Autodesk Inventor part; units mm, degrees
ref_plane "Work Plane1" through (-3.0381, -3.0381, 30.2492) normal (0, 0, -1) x (0, 1, 0)
ref_plane "Work Plane2" through (-3.0898, -3.0898, 32.8492) normal (0, 0, -1) x (0.0301, 0.9995, 0)
ref_plane "YZ Plane" through (0, 0, 0) normal (1, 0, 0) x (0, 1, 0)
sketch "Sketch2" plane through (0, 0, 0) normal (0, 0, 1) x (1, 0, 0)
  circle A0 centre (0, 0) radius 3
  dimension "d0" = 6
ref_plane "Work Plane1" through (-3.0381, -3.0381, 30.2492) normal (0, 0, -1) x (0, 1, 0)
ref_plane "Work Plane2" through (-3.0898, -3.0898, 32.8492) normal (0, 0, -1) x (0.0301, 0.9995, 0)
extrude "Extrusion1" add sketch "Sketch2" along normal up to surface (32.8492 mm away)
sketch "Sketch3" plane through (0, 0, 32.8492) normal (0, 0, 1) x (1, 0, 0)
  point P0 (0, 0)
  point P1 (0, 0)
hole "Hole1" at (0, 0, 32.8492) direction (0, 0, -1) diameter 3.242 depth 10
sketch "Sketch4" plane through (0, 0, 0) normal (0, 0, -1) x (-1, 0, 0)
  circle A0 centre (0, 0) radius 1.621
  point P0 (0, 0)
hole "Hole2" at (0, 0, 0) direction (0, 0, 1) diameter 3.242 depth 10
properties part number "GEARBOX STANDOFFS"
For this review, take the finished solid that the model builds, in its own axes (mm). A direction names the side the tool comes from. Coordinates: 2 decimals unless noted, no trailing zeros. Order: outer loops, then holes, each group sorted by start corner. A loop starts at its lowest first (then second) coordinate and runs counter-clockwise, first axis right, second up. Notation, with made-up numbers: (-25, 77) -> (17, 77) arc R9 ccw to (17, 89) -> close; hole circle Ø5 at (81, -21.5). An arc over 180 degrees is marked (long way). Use CSV: the item, a comma, the result in double quotes. Start each with the question number.
Item 1: Draft analysis for pull direction Y (two halves, no side actions). For faces 1 (the face through (-3, 0, 16)), 2 (the face through (1.3, -1.3, 32.849)), 3 (the face through (1.438, 0.748, 5.07)), state which applies: pulls with the +Y half, pulls with the -Y half, needs draft (parallel to the pull), parting line crosses it, or undercut.
Item 2: Insertion check: pin 1 (1 mm diameter, centred on x = 0.5, y = 0, fed in from -Z); pin 2 (1.5 mm diameter, centred on x = 0.5, y = -0.5, fed in from +Z); pin 3 (1 mm diameter, centred on y = -1.5, z = 12.5, fed in from -X). Each pin has a flat end and moves straight along its axis. Give the tip position at first contact, or say it passes through.
Item 3: We need section C-C, the plane z = 8. Give the boundary of the cut face in (x, y).
Item 4: We need section A-A, the plane y = 0. Give the boundary of the cut face in (x, z), then the cut area to 3 significant figures.
Item 5: For faces 4 (the face through (1.3, -1.3, 0)), 5 (the face through (1.438, -0.748, 27.779)), 6 (the face through (0, 0, 10)), list the 3-axis set-ups (+Z, -Z, +X, -X, +Y, -Y) from which the entire face can be reached by the end or side of a thin tool; tool diameter is ignored.
Item 6: Wall thickness on probe 1 along X at (y, z) = (-0.05, 28.5); probe 2 along Z at (x, y) = (1, 0.75): over which ranges is each line inside the solid? List them lowest first.
Item 7: We need section D-D, the plane x = -2.1. Give the boundary of the cut face in (y, z), then the cut area to 3 significant figures.
Derived:
1,face 1,"parting line crosses it"
1,face 2,"needs draft"
1,face 3,"undercut"
2,pin 1,"stops at z = 10"
2,pin 2,"stops at z = 22.85"
2,pin 3,"stops at x = -2.83"
3,outline,"circle Ø6 at (0, 0); hole circle Ø3.24 at (0, 0)"
4,outline,"(-3, 0) -> (-1.62, 0) -> (-1.62, 10) -> (1.62, 10) -> (1.62, 0) -> (3, 0) -> (3, 32.85) -> (1.62, 32.85) -> (1.62, 22.85) -> (-1.62, 22.85) -> (-1.62, 32.85) -> (-3, 32.85) -> close"
4,area,"132 mm^2"
5,face 4,"-Z, +X, -X, +Y, -Y"
5,face 5,"+Z"
5,face 6,"-Z"
6,probe 1,"x = -3 to -1.62, 1.62 to 3"
6,probe 2,"z = 10 to 22.85"
7,outline,"(-2.14, 0) -> (2.14, 0) -> (2.14, 32.85) -> (-2.14, 32.85) -> close"
7,area,"141 mm^2"
